Could you check a few things on this model? Use its own coordinates, in mm. A direction names the side the tool comes from. Give positions to 0.01 mm unless a question says otherwise; leave off trailing zeros. Order: outer loops, then holes, each group sorted by start corner. A loop starts at its lowest first (then second) coordinate and runs counter-clockwise, first axis right, second up.
Autodesk Inventor part; units mm, degrees
ref_plane "YZ Plane" through (0, 0, 0) normal (1, 0, 0) x (0, 1, 0)
ref_plane "XZ Plane" through (0, 0, 0) normal (0, 1, 0) x (-1, 0, 0)
ref_plane "XY Plane" through (0, 0, 0) normal (0, 0, 1) x (1, 0, 0)
sketch "Sketch1" plane through (0, 0, 0) normal (1, 0, 0) x (0, 1, 0)
  line L0 (0, -2) -> (4, -2)
  line L1 (4, -2) -> (4, -3)
  line L2 (4, -3) -> (0.5972, -3.6)
  line L3 (0, -3.6) -> (0, -2)
  line L4 (-4, 0) -> (24, 0)
  line L5 (0, -3.6) -> (0.5972, -3.6)
  line L6 (4, -2) -> (8, -2)
  line L7 (8, -2) -> (8, -3)
  line L8 (8, -3) -> (4.5972, -3.6)
  line L9 (4, -3.6) -> (4, -2)
  line L10 (4, -3.6) -> (4.5972, -3.6)
  line L11 (8, -2) -> (12, -2)
  line L12 (12, -2) -> (12, -3)
  line L13 (12, -3) -> (8.5972, -3.6)
  line L14 (8, -3.6) -> (8, -2)
  line L15 (8, -3.6) -> (8.5972, -3.6)
  line L16 (12, -2) -> (16, -2)
  line L17 (16, -2) -> (16, -3)
  line L18 (16, -3) -> (12.5972, -3.6)
  line L19 (12, -3.6) -> (12, -2)
  line L20 (12, -3.6) -> (12.5972, -3.6)
  line L21 (16, -2) -> (20, -2)
  line L22 (20, -2) -> (20, -3)
  line L23 (20, -3) -> (16.5972, -3.6)
  line L24 (16, -3.6) -> (16, -2)
  line L25 (16, -3.6) -> (16.5972, -3.6)
  point P0 (0, 0)
  dimension "d0" = 1
  dimension "d1" = 2
  dimension "d2" = 4
  dimension "d3" = 10
  dimension "d4" = 0
  dimension "d12" = 3.6
  dimension "d15" = 4
revolve "Revolution1" add sketch "Sketch1" angle 360 about axis through (0, -10, 0) along (0, 1, 0)
sketch "Sketch2" plane through (0, 0, 0) normal (1, 0, 0) x (0, 1, 0)
  line L0 (0, -3.6) -> (0, 3.6)
  line L1 (20, -2) -> (20, 2)
  line L2 (0, -3.6) -> (20, -3.6)
  line L3 (20, -3.6) -> (20, -2)
  line L4 (20, -2) -> (0, -2)
  line L5 (0, -2) -> (0, -3.6)
  line L6 (0, 3.6) -> (20, 3.6)
  line L7 (20, 3.6) -> (20, 2)
  line L8 (20, 2) -> (0, 2)
  line L9 (0, 2) -> (0, 3.6)
  point P0 (0, 0)
  point P1 (0, 1.6227)
  point P2 (20, -3.8756)
  dimension "d24" = 1.6
extrude "Extrusion1" add sketch "Sketch2" along normal blind 3.7 contours L0 L4 L3 L2 | L0 L6 L7 L8
properties part number "nipple"
Item 1: For faces 4 (the flat face through (3.2, 16, 0)), 5 (the flat face through (3.7, 10, -3)), 6 (the conical face through (-3.237, 10.653, 0.071)), which set-ups out of +Z, -Z, +X, -X, +Y, -Y let a thin tool reach every point of the face, with its end or its side?
Findings:
face 4: +X
face 5: +Z, -Z, +X, +Y, -Y
face 6: -X
Item 2: Imagine slicing it at B-B on y = 8.25. List the corners of the cut face in (x, z) for me, then the cut area to 3 significant figures.
Findings:
outline: (0, -3.6) - (3.7, -3.6) - (3.7, -2) - (2.99, -2) arc R3.6 ccw to (2.99, 2) - (3.7, 2) - (3.7, 3.6) - (0, 3.6) arc R3.6 ccw to start; hole circle Ø4 at (0, 0)
area: 33.3 mm2
Item 3: Imagine slicing it at C-C on x = 0.5. List the corners of the cut face in (y, z) for me.
Findings:
outline: (0, -3.6) - (20, -3.6) - (20, -1.94) - (0, -1.94) - close; (0, 1.94) - (20, 1.94) - (20, 3.6) - (0, 3.6) - close
Item 4: Imagine slicing it at D-D on x = 2.75. Give the number of separate pieces and of enclosed holes in the cut face, then the cut area to 3 significant figures.
Findings:
separate pieces: 1
enclosed holes: 8
area: 135 mm2
Item 5: We'd pull the mould along Z, two halves only. Please class faces 1 (the flat face through (-3, 8, -1)), 2 (the conical face through (3.3, 10.3, 0)), 3 (the cylindrical face through (-3.6, 12.3, -0.1)): +Z half, -Z half, draft (parallel to the pull), parting line (faces both ways), or undercut.
Findings:
face 1: draft
face 2: undercut
face 3: parting line
Item 6: For pin 1 (0.7 mm diameter, centred on y = 1.5, z = 3, fed in from -X); pin 2 (1.1 mm diameter, centred on x = -1, z = -0.5, fed in from -Y); pin 3 (0.5 mm diameter, centred on y = 10, z = 3, fed in from -X), each with a flat end and sliding along its axis, tell me the tip position at first contact or that it passes through.
Findings:
pin 1: stops at x = -2.21
pin 2: passes through
pin 3: stops at x = -1.93
